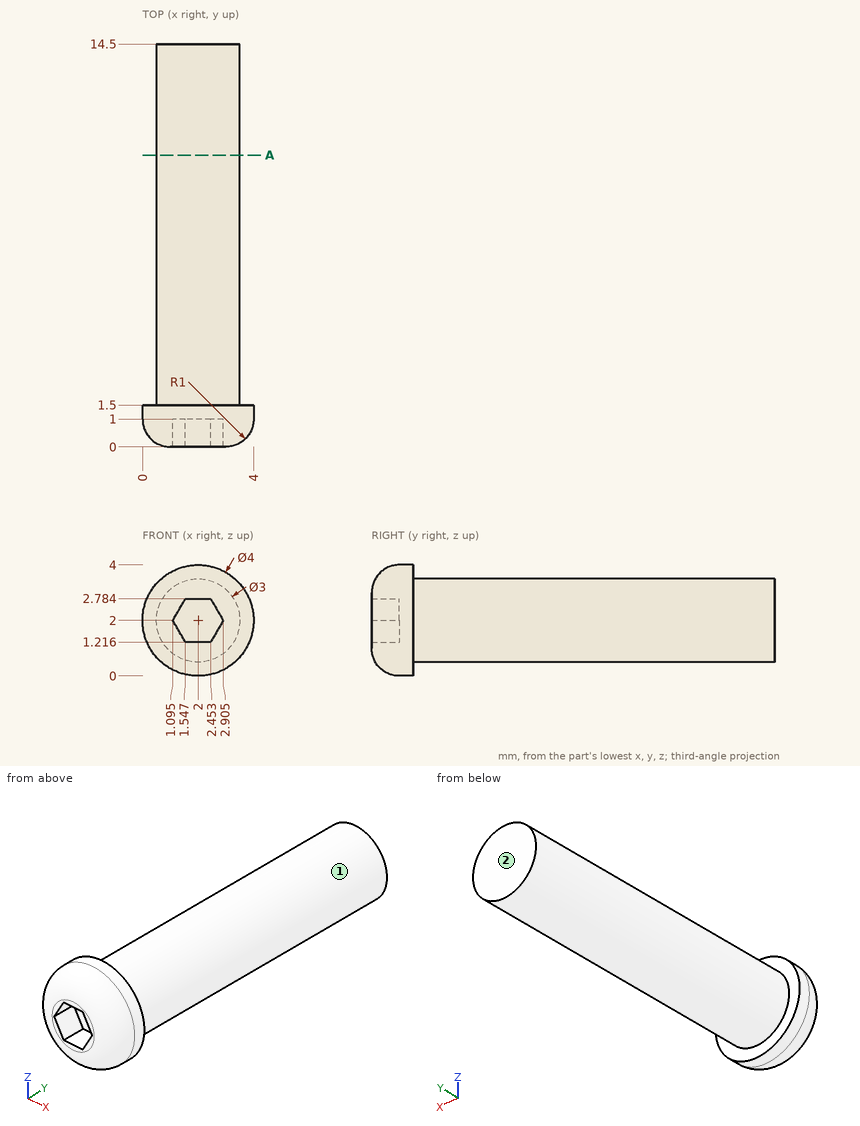
Verification items for this drawing (mm, ordinates from the low corner). Give positions to 0.01 mm unless a question says otherwise; leave off trailing zeros. Write each loop counter-clockwise with the first axis right and the second up, starting at its lowest first coordinate (ties: lowest second). Pieces come first, ordered by that corner, then holes. Notation, with made-up numbers: (15, 85.25) -> (72, 85.25) arc R10 cw to (72, 101.25) -> close; hole circle Ø5 at (-12, 55). An arc over 180 degrees is marked (long way). Use one line per item in the form item = value.
Item 1: Scan lines: line 1 (Y direction, x = 2.25, z = 1.35); line 2 (Z direction, x = 2.05, y = 11.25). Record each from-to range of solid material in increasing order.
Results list:
line_1 = 1 to 14.5
line_2 = 0.5 to 3.5
Item 2: Mould release check, pull along Y, two halves, no side actions. Record for the marked faces 1 and 2: released by +Y, released by -Y, zero draft, split by the parting line, or undercut.
Results list:
face_1 = zero draft
face_2 = released by +Y
Item 3: Depth check by flat-ended pin: pin 1 Ø1.5 at (y, z) = (5.5, 2.5) entering from +X; pin 2 Ø0.7 at (x, y) = (2, 0.5) entering from +Z. Enter the tip coordinate at first touch or a pass-through.
Results list:
pin_1 = 3.5
pin_2 = 3.99
Item 4: Sectioned sample at A-A on y = 10.5. Enter the section's corners in (x, z).
Results list:
outline = circle Ø3 at (2, 2)
